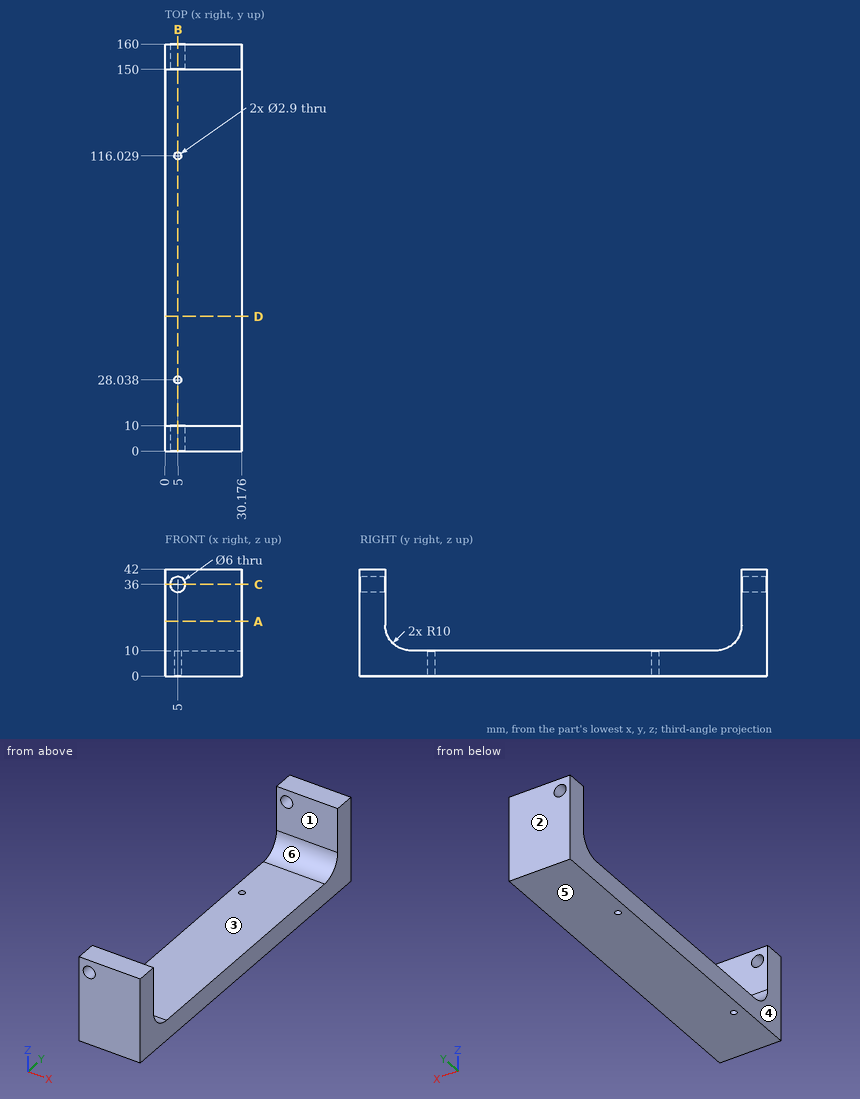
For this review, use the dimensioned drawing (mm, ordinates from the lowest corner) and the shaded views. A direction names the side the tool comes from. Coordinates: 2 decimals unless noted, no trailing zeros. Loops run counter-clockwise (first coordinate to the right, second up) from the corner with the lowest first, then second, coordinate; pieces in that order, holes last. Notation, with made-up numbers: (-37.75, 50.25) -> (-27.75, 50.25) arc R31 cw to (-27.75, 75.25) -> close; hole circle Ø11 at (74, 26.25). An arc over 180 degrees is marked (long way). Use a Markdown table: item, result. Add a question column.
Item 1: Clearance check with flat-ended pins moving along their axes: P1, Ø8, axis at x = 5, z = 36, coming from the -Y side; P2, Ø3.5, axis at x = 5, z = 36, coming from the -Y side; P3, Ø15, axis at x = 16.5, y = 50.5, coming from the +Z side. State where each tip first meets the part, or that it passes through.
Item 2: Machinability: for the marked faces 5 and 6, which of the approach directions +Z, -Z, +X, -X, +Y, -Y give a long, thin tool a straight path to every point of the face, cutting with its end or side? Answer none if there is none.
Item 3: We need section B-B, the plane x = 5. Write out the cut boundary in (y, z).
Item 4: Wall thickness on L1, parallel to Y at x = 5, z = 7; L2, parallel to Y at x = 3, z = 33; L3, parallel to Z at x = 19, y = 83.5: over which ranges is each line inside the solid? List them lowest first. Write a range as from..to.
Item 5: The part is to be moulded in two halves that separate along Y. For the marked faces 1, 2, 3 and 4, say which applies: +Y half, -Y half, draft (parallel to the pull), parting line (faces both ways), or undercut.
Item 6: We need section C-C, the plane z = 36. Write out the cut boundary in (x, y).
Item 7: We need section A-A, the plane z = 21.5. Write out the cut boundary in (x, y).
Item 8: We need section D-D, the plane y = 53. Write out the cut boundary in (x, z).
Numbers:
| question | item | result |
|---|---|---|
| 1 | P1 | stops at y = 0 |
| 1 | P2 | passes through |
| 1 | P3 | stops at z = 10 |
| 2 | face 5 | -Z, +X, -X, +Y, -Y |
| 2 | face 6 | +Z, +X, -X |
| 3 | outline | (0, 0) -> (26.59, 0) -> (26.59, 10) -> (20, 10) arc R10 cw to (10, 20) -> (10, 33) -> (0, 33) -> close; (0, 39) -> (10, 39) -> (10, 42) -> (0, 42) -> close; (29.49, 0) -> (114.58, 0) -> (114.58, 10) -> (29.49, 10) -> close; (117.48, 0) -> (160, 0) -> (160, 33) -> (150, 33) -> (150, 20) arc R10 cw to (140, 10) -> (117.48, 10) -> close; (150, 39) -> (160, 39) -> (160, 42) -> (150, 42) -> close |
| 4 | L1 | y = 0..26.59, 29.49..114.58, 117.48..160 |
| 4 | L2 | y = 0..10, 150..160 |
| 4 | L3 | z = 0..10 |
| 5 | face 1 | undercut |
| 5 | face 2 | +Y half |
| 5 | face 3 | undercut |
| 5 | face 4 | draft |
| 6 | outline | (0, 0) -> (2, 0) -> (2, 10) -> (0, 10) -> close; (0, 150) -> (2, 150) -> (2, 160) -> (0, 160) -> close; (8, 0) -> (30.18, 0) -> (30.18, 10) -> (8, 10) -> close; (8, 150) -> (30.18, 150) -> (30.18, 160) -> (8, 160) -> close |
| 7 | outline | (0, 0) -> (30.18, 0) -> (30.18, 10) -> (0, 10) -> close; (0, 150) -> (30.18, 150) -> (30.18, 160) -> (0, 160) -> close |
| 8 | outline | (0, 0) -> (30.18, 0) -> (30.18, 10) -> (0, 10) -> close |
